from build123d import *

# Parameters (mm, degrees)
F1_DEPTH = 152.4
F2_R     = 5.08


# Not quite as in the source:
# - two fillets or chamfers of one size are made in one step
# - a feature names something its author has since deleted; it is built from what else it names


with BuildPart() as f1:
    # F0 (on Front) → F1 (new body)
    with BuildSketch(Plane.XZ):
        with BuildLine():
            Line((228.6, -38.1), (228.6, 0))
            ThreePointArc((228.6, 0), (195.1223050896, 80.8223050896), (114.3, 114.3))
            ThreePointArc((114.3, 114.3), (33.4776949104, 80.8223050896), (0, 0))
            Line((0, 0), (0, -38.1))
            Line((0, -38.1), (12.7, -38.1))
            Line((12.7, -38.1), (12.7, 0))
            ThreePointArc((12.7, 0), (114.3, 101.6), (215.9, 0))
            Line((215.9, 0), (215.9, -38.1))
            Line((215.9, -38.1), (228.6, -38.1))
        make_face()
        with BuildLine():
            ThreePointArc((114.3, 114.3), (195.1223050896, 80.8223050896), (228.6, 0))
            Line((228.6, 0), (228.6, 114.3))
            Line((228.6, 114.3), (114.3, 114.3))
        make_face()
        with BuildLine():
            ThreePointArc((0, 0), (33.4776949104, 80.8223050896), (114.3, 114.3))
            Line((114.3, 114.3), (0, 114.3))
            Line((0, 114.3), (0, 0))
        make_face()
    extrude(amount=F1_DEPTH)

    # F2
    f2_edges = [f1.edges().sort_by_distance(p)[0] for p in [
        (114.3, -152.4, 101.6),
        (114.3, 0, 101.6),
        (222.25, -152.4, -38.1),
        (6.35, -152.4, -38.1),
        (12.7, -76.2, -38.1),
        (0, -76.2, -38.1),
        (6.35, 0, -38.1),
        (215.9, -76.2, -38.1),
        (215.9, 0, -19.05),
        (215.9, -152.4, -19.05),
        (228.6, -76.2, -38.1),
        (228.6, 0, 38.1),
        (228.6, -152.4, 38.1),
        (114.3, -152.4, 114.3),
        (0, -152.4, 38.1),
        (12.7, 0, -19.05),
        (12.7, -152.4, -19.05),
    ]]
    fillet(f2_edges, radius=F2_R)


solid = f1.part
Could you check a few things on this model? Use its own coordinates, in mm. A direction names the side the tool comes from. Coordinates: 2 decimals unless noted, no trailing zeros. Order: outer loops, then holes, each group sorted by start corner. A loop starts at its lowest first (then second) coordinate and runs counter-clockwise, first axis right, second up. Notation, with made-up numbers: (-24.5, 71) -> (-0.5, 71) arc R8 ccw to (-0.5, 77) -> close; hole circle Ø5 at (59.25, 75). An arc over 180 degrees is marked (long way). One line per item, written item: value. Start each with the question number.
1) Imagine slicing it at A-A on y = -46. List the corners of the cut face in (x, z) for me, plus the area to 3 significant figures.
2) I'm going to push flat-ended pins straight in: pin 1 (4 mm diameter, centred on x = 73, z = 93, fed in from +Y); pin 2 (12 mm diameter, centred on x = 154, y = -83, fed in from -Z); pin 3 (4 mm diameter, centred on x = 138, y = -55.5, fed in from -Z). Where does each tip first touch, or does it pass through?
3) If I drill on L1, parallel to X at y = -122, z = 2.5; L2, parallel to X at y = -80.5, z = 72.5; L3, parallel to Z at x = 165, y = -65.5, over which ranges is the centre line in solid material (lowest first)? Write a range as [from, to].
4) We'd pull the mould along X, two halves only. Please class faces 6 (the flat face through (228.6, -75, 40)), 7 (the cylindrical face through (217.349, -74.691, -36.572)), 8 (the cylindrical face through (1.449, -74.691, -36.572)): +X half, -X half, draft (parallel to the pull), parting line (faces both ways), or undercut.
5) Which directions (+Z, -Z, +X, -X, +Y, -Y) give clear straight access to the entire face, cutting with the end or side of a thin tool? Please do faces 1 (the cylindrical face through (4.71, -0.95, -35.98)), 2 (the cylindrical face through (11.251, -1.528, -16.279)), 3 (the cylindrical face through (1.449, -150.872, 39.609)), 4 (the flat face through (215.9, -75, -16)), 5 (the cylindrical face through (217.349, -150.872, -16.741)).
Answer list:
1. outline: (0, -33.02) arc R5.08 ccw to (5.08, -38.1) -> (7.62, -38.1) arc R5.08 ccw to (12.7, -33.02) -> (12.7, 0) arc R101.6 cw to (215.9, 0) -> (215.9, -33.02) arc R5.08 ccw to (220.98, -38.1) -> (223.52, -38.1) arc R5.08 ccw to (228.6, -33.02) -> (228.6, 114.3) -> (0, 114.3) -> close
1. area: 10,900 mm2
2. pin 1: stops at y = -0.92
2. pin 2: stops at z = 90.74
2. pin 3: stops at z = 98.3
3. L1: x = [0, 12.73], [215.87, 228.6]
3. L2: x = [0, 43.12], [185.48, 228.6]
3. L3: z = [88.05, 114.3]
4. face 6: +X half
4. face 7: undercut
4. face 8: -X half
5. face 1: -Z, -X, +Y
5. face 2: -Z, +Y
5. face 3: +Z, -Z, -X, -Y
5. face 4: -Z, +Y, -Y
5. face 5: -Z, -Y
